from build123d import *

# Parameters (mm, degrees)
SKETCH_1_R          = 1.5
EXTRUDE_1_DEPTH     = 10
SKETCH_2_R          = 1.75
CUT_EXTRUDE_1_DEPTH = 15.568802284
FILLET_2_R          = 4


with BuildPart() as part:
    # Эскиз1 → Бобышка-Вытянуть1 (new body)
    with BuildSketch(Plane(origin=(0, 0, 0), x_dir=(0, 0, -1), z_dir=(1, 0, 0))):
        with BuildLine():
            Line((-10, -3), (10, -3))
            Line((10, -3), (10, 0))
            Line((10, 0), (3.5, 0))
            ThreePointArc((3.5, 0), (0, 3.5), (-3.5, 0))
            Line((-3.5, 0), (-10, 0))
            Line((-10, 0), (-10, -3))
        make_face()
        Circle(SKETCH_1_R, mode=Mode.SUBTRACT)
    extrude(amount=EXTRUDE_1_DEPTH)

    # Эскиз2 → Вырез-Вытянуть1 (cut, through all)
    with BuildSketch(Plane(origin=(0, 0, 0), x_dir=(1, 0, 0), z_dir=(0, 1, 0))):
        with Locations(Location((5, 6.75, 0), (0, 0, 270))):
            Circle(SKETCH_2_R)
        with Locations(Location((5, -6.75, 0), (0, 0, 270))):
            Circle(SKETCH_2_R)
    extrude(amount=-CUT_EXTRUDE_1_DEPTH, mode=Mode.SUBTRACT)

    # Скругление2
    fillet_2_edges = [part.edges().sort_by_distance(p)[0] for p in [
        (10, -1.5, -10),
        (10, -1.5, 10),
        (0, -1.5, -10),
        (0, -1.5, 10),
    ]]
    fillet(fillet_2_edges, radius=FILLET_2_R)


solid = part.part
Check sheet for the modelled part. Datum: model origin and axes. Units: mm. A direction names the side the tool comes from. Round coordinates to 2 decimals unless told otherwise and drop trailing zeros. Loops run counter-clockwise (first coordinate to the right, second up) from the corner with the lowest first, then second, coordinate; pieces in that order, holes last. Notation, with made-up numbers: M -22,30.5 L 31,30.5 A13 ccw 31,37.5 Z; hole C -16,-32.75 d4. An arc over 180 degrees is marked long. One line per item, written item: value.
(1) Sectioned sample at C-C, the plane x = 4.5. Record the cut outline in (y, z).
Computed values:
outline: M -3,-10 L 0,-10 L 0,-8.43 L -3,-8.43 Z; M -3,-5.07 L 0,-5.07 L 0,-3.5 A3.5 ccw 0,3.5 L 0,5.07 L -3,5.07 Z; M -3,8.43 L 0,8.43 L 0,10 L -3,10 Z; hole C 0,0 d3
(2) Sectioned sample at B-B, the plane y = -1. Record the cut outline in (x, z), then the cut area to 3 significant figures.
Computed values:
outline: M 0,-6 A4 ccw 4,-10 L 6,-10 A4 ccw 10,-6 L 10,-1.12 L 0,-1.12 Z; M 0,1.12 L 10,1.12 L 10,6 A4 ccw 6,10 L 4,10 A4 ccw 0,6 Z; hole C 5,-6.75 d3.5; hole C 5,6.75 d3.5
area: 145 mm^2
(3) Sectioned sample at D-D, the plane x = 7.5. Record the cut outline in (y, z).
Computed values:
outline: M -3,-9.71 L 0,-9.71 L 0,-3.5 A3.5 ccw 0,3.5 L 0,9.71 L -3,9.71 Z; hole C 0,0 d3
(4) Thickness scan on line 1 (Z direction, x = 4.25, y = -2.5); line 2 (Y direction, x = 6.75, z = 8); line 3 (Y direction, x = 7.75, z = 0). Record the ranges inside material, lowest first.
Computed values:
line 1: z = -10 to -8.33, -5.17 to 5.17, 8.33 to 10
line 2: y = -3 to 0
line 3: y = -3 to -1.5, 1.5 to 3.5
(5) Depth check by flat-ended pin: pin 1 Ø4 at (x, z) = (8, 3) entering from +Y; pin 2 Ø1 at (x, y) = (1, 2.5) entering from +Z; pin 3 Ø2 at (x, z) = (6.5, -7.5) entering from +Y; pin 4 Ø3 at (x, z) = (5, 6.75) entering from -Y. Enter the tip coordinate at first touch or a pass-through.
Computed values:
pin 1: stops at y = 3.35
pin 2: stops at z = 2.87
pin 3: stops at y = 0
pin 4: passes through
(6) Release check for a two-part mould opening along Y. For faces 3 (the face through (4.93, 0.07, 1.5)), 4 (the face through (0, -2, 0)), 5 (the face through (4, 0, 5)) record: +Y half, -Y half, draft (parallel to the pull), parting line (faces both ways), or undercut.
Computed values:
face 3: undercut
face 4: draft
face 5: +Y half
(7) Sectioned sample at A-A, the plane z = 0. Record the cut outline in (x, y), then the cut area to 3 significant figures.
Computed values:
outline: M 0,-3 L 10,-3 L 10,-1.5 L 0,-1.5 Z; M 0,1.5 L 10,1.5 L 10,3.5 L 0,3.5 Z
area: 35.0 mm^2
(8) Access from +Z, -Z, +X, -X, +Y, -Y to the whole of each face (thin tool, end or side, straight path). Record for faces 1 (the face through (4, 0, -5)), 2 (the face through (8.797, -1.521, 8.859)).
Computed values:
face 1: -Z, +X, -X, +Y
face 2: +Z, +X, +Y, -Y
